Verification items for the finished model (mm, model axes). Face numbers are marked on the shaded views. A direction names the side the tool comes from. Coordinates: 2 decimals unless noted, no trailing zeros. Write each loop counter-clockwise with the first axis right and the second up, starting at its lowest first coordinate (ties: lowest second). Pieces come first, ordered by that corner, then holes. Notation, with made-up numbers: (-18.5, 19.5) -> (17.5, 19.5) arc R14 cw to (17.5, 41.5) -> close; hole circle Ø4 at (37.5, 44.5). An arc over 180 degrees is marked (long way). Write item = value, one per line. Start each with the question number.
(1) Set-up check for the marked faces 4, 5 and 6: record each of +Z, -Z, +X, -X, +Y, -Y from which the full face is reachable in a straight line by a thin tool's end or side.
(2) Gauge pin test, flat ends, axial feed: pin 1 Ø5.5 at (y, z) = (0, 0) entering from +X; pin 2 Ø2.5 at (x, y) = (3.5, 7) entering from -Z; pin 3 Ø4 at (y, z) = (-1.5, -3) entering from -X; pin 4 Ø4 at (x, y) = (4.5, 10.09) entering from +Z. Record the tip position at first contact, or that the pin passes through.
(3) Section check A-A (y = 0). Record the cut outline in (x, z), plus the area to 3 significant figures.
(4) Section check B-B (z = -2.5). Record the cut outline in (x, y), plus the area to 3 significant figures.
(5) Material ranges on probe 1 along Z at (x, y) = (0.5, 7); probe 2 along X at (y, z) = (10, 4.5); probe 3 along Y at (x, z) = (4.5, 1.75), recorded low to high. Write a range as [from, to].
(6) Section check D-D (x = 7.25). Record the cut outline in (y, z), plus the area to 3 significant figures.
(7) Section check C-C (x = 5.25). Record the cut outline in (y, z).
(8) Mould release check, pull along X, two halves, no side actions. Record for the marked faces 1, 2 and 3: released by +X, released by -X, zero draft, split by the parting line, or undercut.
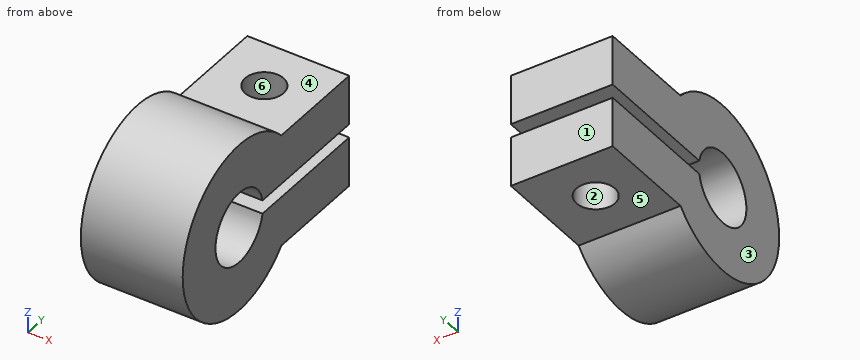
Autodesk Inventor part; units mm, degrees
ref_plane "YZ Plane" through (0, 0, 0) normal (1, 0, 0) x (0, 1, 0)
ref_plane "XZ Plane" through (0, 0, 0) normal (0, 1, 0) x (-1, 0, 0)
ref_plane "XY Plane" through (0, 0, 0) normal (0, 0, 1) x (1, 0, 0)
sketch "スケッチ1" plane through (0, 0, 0) normal (1, 0, 0) x (0, 1, 0)
  circle A0 centre (0, 0) radius 3.15
  circle A1 centre (0, 0) radius 7.5
  line L0 (0, 0) -> (14.5902, 0)
  line L1 (14.5902, 5) -> (5.5902, 5)
  line L2 (5.5902, 5) -> (5.5902, -5)
  line L3 (5.5902, -5) -> (14.5902, -5)
  line L4 (14.5902, -5) -> (14.5902, 5)
  line L5 (14.5902, 0.6) -> (5.5902, 0.6)
  line L6 (5.5902, 0.6) -> (5.5902, -0.6)
  line L7 (5.5902, -0.6) -> (14.5902, -0.6)
  line L8 (14.5902, -0.6) -> (14.5902, 0.6)
  line L9 (5.5902, 0.6) -> (3.0923, 0.6)
  line L10 (5.5902, -0.6) -> (3.0923, -0.6)
  dimension "d1" = 15
  dimension "d0" = 6.3
  dimension "d2" = 1.2
  dimension "d3" = 9
  dimension "d4" = 10
extrude "押し出し1" add sketch "スケッチ1" along normal blind 9 contours A0 L10 L2 A1 L9 | L2 A1 L5 | L7 A1 L2 | L1 L4 L5 A1 | A1 L7 L4 L3
sketch "スケッチ2" plane through (0, 5.5902, -5) normal (0, 0, -1) x (-1, 0, 0)
  line L0 (0, 9) -> (-9, 9)
  line L1 (-4.5, 9) -> (-4.5, 3.2578)
  point P0 (0, -5.5902)
  point P1 (-4.5, 4.5)
  dimension "d7" = 4.5
hole "穴1" at (4.5, 10.0902, -5) direction (0, 0, 1) diameter 3.4 end through all
properties part number "SetCollar_d6"
Response:
q1.face_4 = +Z, +X, -X, +Y
q1.face_5 = -Z, +X, -X, +Y
q1.face_6 = +Z, -Z
q2.pin_1 = through
q2.pin_2 = -5
q2.pin_3 = 0
q2.pin_4 = 5
q3.outline = (0, -7.5) -> (9, -7.5) -> (9, -3.15) -> (0, -3.15) -> close; (0, 3.15) -> (9, 3.15) -> (9, 7.5) -> (0, 7.5) -> close
q3.area = 78.3 mm2
q4.outline = (0, -7.07) -> (9, -7.07) -> (9, -1.92) -> (0, -1.92) -> close; (0, 1.92) -> (9, 1.92) -> (9, 14.59) -> (0, 14.59) -> close; hole circle Ø3.4 at (4.5, 10.09)
q4.area = 151 mm2
q5.probe_1 = [-5, -0.6], [0.6, 5]
q5.probe_2 = [0, 2.8], [6.2, 9]
q5.probe_3 = [-7.29, -2.62], [2.62, 8.39], [11.79, 14.59]
q6.outline = (3.09, -0.6) arc R3.15 cw (long way) to (3.09, 0.6) -> (14.59, 0.6) -> (14.59, 5) -> (5.59, 5) arc R7.5 ccw (long way) to (5.59, -5) -> (14.59, -5) -> (14.59, -0.6) -> close
q6.area = 209 mm2
q7.outline = (3.09, -0.6) arc R3.15 cw (long way) to (3.09, 0.6) -> (8.56, 0.6) -> (8.56, 5) -> (5.59, 5) arc R7.5 ccw (long way) to (5.59, -5) -> (8.56, -5) -> (8.56, -0.6) -> close; (11.62, -5) -> (14.59, -5) -> (14.59, -0.6) -> (11.62, -0.6) -> close; (11.62, 0.6) -> (14.59, 0.6) -> (14.59, 5) -> (11.62, 5) -> close
q8.face_1 = zero draft
q8.face_2 = undercut
q8.face_3 = released by -X
